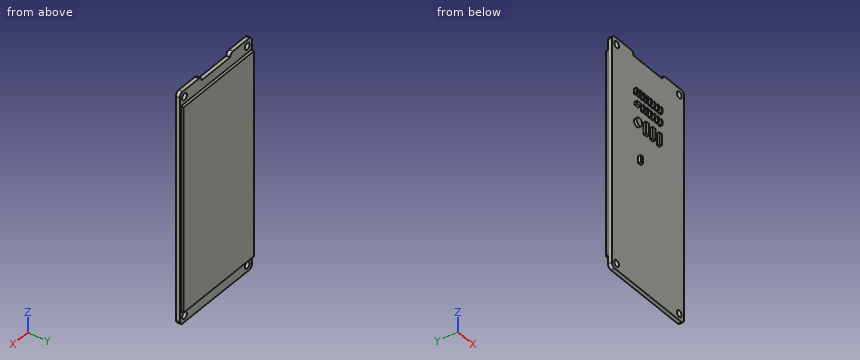
```python
from build123d import *

# Parameters (mm, degrees)
SKETCH1_R           = 1.25
BOSS_EXTRUDE1_DEPTH = 1.5
SKETCH2_W           = 37.118680969
SKETCH2_H           = 79.295382989
BOSS_EXTRUDE2_DEPTH = 1.05
SKETCH3_R           = 1.480960071
SKETCH3_W           = 0.706323155
SKETCH3_H           = 2.007969185
SKETCH3_W_2         = 1.202782264
SKETCH3_H_2         = 2.785488108
SKETCH3_W_3         = 1.512629418
SKETCH3_H_3         = 4.544655772
SKETCH3_W_4         = 1.362329437
SKETCH3_W_5         = 1.179692139
SKETCH3_W_6         = 1.879481301
SKETCH3_H_4         = 1.158224536
BOSS_EXTRUDE3_DEPTH = 1


with BuildPart() as part:
    # Sketch1 → Boss-Extrude1 (new body)
    with BuildSketch(Plane(origin=(0, 0, 0), x_dir=(1, 0, 0), z_dir=(0, 1, 0))):
        with BuildLine():
            Line((1.5, 0), (10, 0))
            ThreePointArc((10, 0), (11.060660172, 0.439339828), (11.5, 1.5))
            Line((11.5, 1.5), (26.5, 1.5))
            ThreePointArc((26.5, 1.5), (26.939339828, 0.439339828), (28, 0))
            Line((28, 0), (36.5, 0))
            ThreePointArc((36.5, 0), (37.560660172, 0.439339828), (38, 1.5))
            Line((38, 1.5), (38, 88))
            ThreePointArc((38, 88), (37.560660172, 89.060660172), (36.5, 89.5))
            Line((36.5, 89.5), (1.5, 89.5))
            ThreePointArc((1.5, 89.5), (0.439339828, 89.060660172), (0, 88))
            Line((0, 88), (0, 1.5))
            ThreePointArc((0, 1.5), (0.439339828, 0.439339828), (1.5, 0))
        make_face()
        with Locations((2.5, 2.5)):
            Circle(SKETCH1_R, mode=Mode.SUBTRACT)
        with Locations((35.5, 2.5)):
            Circle(SKETCH1_R, mode=Mode.SUBTRACT)
        with Locations((35.5, 87)):
            Circle(SKETCH1_R, mode=Mode.SUBTRACT)
        with Locations((2.5, 87)):
            Circle(SKETCH1_R, mode=Mode.SUBTRACT)
    extrude(amount=BOSS_EXTRUDE1_DEPTH)

    # Sketch2 → Boss-Extrude2 (add)
    with BuildSketch(Plane(origin=(0, 1.5, 0), x_dir=(1, 0, 0), z_dir=(0, 1, 0))):
        with Locations((18.880991901, 44.755610098)):
            Rectangle(SKETCH2_W, SKETCH2_H)
    extrude(amount=BOSS_EXTRUDE2_DEPTH)

    # Sketch3 → Boss-Extrude3 (add)
    with BuildSketch(Plane.XZ):
        with Locations((13.144272763, -26.539340378)):
            Circle(SKETCH3_R)
        with Locations((23.149698331, -19.663516122)):
            Rectangle(SKETCH3_W, SKETCH3_H)
        with Locations((14.4411934, -40.235350725)):
            Rectangle(SKETCH3_W_2, SKETCH3_H_2)
        with Locations((17.469755638, -26.538684778)):
            Rectangle(SKETCH3_W_3, SKETCH3_H_3)
        with Locations((20.813975953, -26.538684778)):
            Rectangle(SKETCH3_W_4, SKETCH3_H_3)
        with Locations((24.294071036, -26.538684778)):
            Rectangle(SKETCH3_W_5, SKETCH3_H_3)
        with Locations((24.999698331, -19.663516122)):
            Rectangle(SKETCH3_W, SKETCH3_H)
        with Locations((21.299698331, -19.663516122)):
            Rectangle(SKETCH3_W, SKETCH3_H)
        with Locations((19.449698331, -19.663516122)):
            Rectangle(SKETCH3_W, SKETCH3_H)
        with Locations((17.599698331, -19.663516122)):
            Rectangle(SKETCH3_W, SKETCH3_H)
        with Locations((15.749698331, -19.663516122)):
            Rectangle(SKETCH3_W, SKETCH3_H)
        with Locations((12.900061618, -19.576771436)):
            Rectangle(SKETCH3_W_6, SKETCH3_H_4)
        with Locations((23.149698331, -15.063516122)):
            Rectangle(SKETCH3_W, SKETCH3_H)
        with Locations((21.299698331, -15.063516122)):
            Rectangle(SKETCH3_W, SKETCH3_H)
        with Locations((19.449698331, -15.063516122)):
            Rectangle(SKETCH3_W, SKETCH3_H)
        with Locations((17.599698331, -15.063516122)):
            Rectangle(SKETCH3_W, SKETCH3_H)
        with Locations((15.749698331, -15.063516122)):
            Rectangle(SKETCH3_W, SKETCH3_H)
        with Locations((13.899698331, -15.063516122)):
            Rectangle(SKETCH3_W, SKETCH3_H)
        with Locations((12.049698331, -15.063516122)):
            Rectangle(SKETCH3_W, SKETCH3_H)
        with Locations((24.999698331, -15.063516122)):
            Rectangle(SKETCH3_W, SKETCH3_H)
    extrude(amount=BOSS_EXTRUDE3_DEPTH)


solid = part.part
```
The listing builds one solid part. Answer for the finished solid, in the listing's coordinates (mm). Coordinates: 2 decimals unless noted, no trailing zeros. Write each loop counter-clockwise with the first axis right and the second up, starting at its lowest first coordinate (ties: lowest second). Pieces come first, ordered by that corner, then holes. Notation, with made-up numbers: (-11, 73.5) - (44, 73.5) arc R23 ccw to (44, 87.5) - close; hole circle Ø5 at (9, -20.75). An arc over 180 degrees is marked (long way). Return JSON: item names as keys, results as strings. Group by question number.
Q1. Find the intervals of material crossed by line 1 along X through (y, z) = (0.65, -87); line 2 along Z through (x, y) = (2.5, 0.3); line 3 along X through (y, z) = (-0.5, -27), in increasing order. Write a range as [from, to].
Q2. The part is cut by section A-A on x = 35.5. Write down the section's boundary in (y, z).
Q3. Flat-ended cylindrical pins translate along their axes: pin 1 Ø0.5 at (y, z) = (-0.5, -20) entering from +X; pin 2 Ø3 at (x, z) = (22.5, -11) entering from -Y; pin 3 Ø0.6 at (x, y) = (21.5, -0.5) entering from +Z. Find the tip coordinate at first contact, or state that the pin passes through.
Q4. The part is cut by section C-C on z = -33.5. Write down the section's boundary in (x, y), and give its area (3 significant figures).
Q5. The part is cut by section B-B on z = -87. Write down the section's boundary in (x, y), and give its area (3 significant figures).
Evaluation:
{
 "1": {"line 1": "x = [0, 1.25], [3.75, 34.25], [36.75, 38]", "line 2": "z = [-89.5, -88.25], [-85.75, -3.75], [-1.25, 0]", "line 3": "x = [11.74, 14.55], [16.71, 18.23], [20.13, 21.5], [23.7, 24.88]"},
 "2": {"outline": "(0, -89.5) - (1.5, -89.5) - (1.5, -88.25) - (0, -88.25) - close; (0, -85.75) - (1.5, -85.75) - (1.5, -84.4) - (2.55, -84.4) - (2.55, -5.11) - (1.5, -5.11) - (1.5, -3.75) - (0, -3.75) - close; (0, -1.25) - (1.5, -1.25) - (1.5, 0) - (0, 0) - close"},
 "3": {"pin 1": "stops at x = 25.35", "pin 2": "stops at y = 0", "pin 3": "stops at z = -14.06"},
 "4": {"outline": "(0, 0) - (38, 0) - (38, 1.5) - (37.44, 1.5) - (37.44, 2.55) - (0.32, 2.55) - (0.32, 1.5) - (0, 1.5) - close", "area": "96.0 mm2"},
 "5": {"outline": "(0, 0) - (1.25, 0) - (1.25, 1.5) - (0, 1.5) - close; (3.75, 0) - (34.25, 0) - (34.25, 1.5) - (3.75, 1.5) - close; (36.75, 0) - (38, 0) - (38, 1.5) - (36.75, 1.5) - close", "area": "49.5 mm2"}
}
